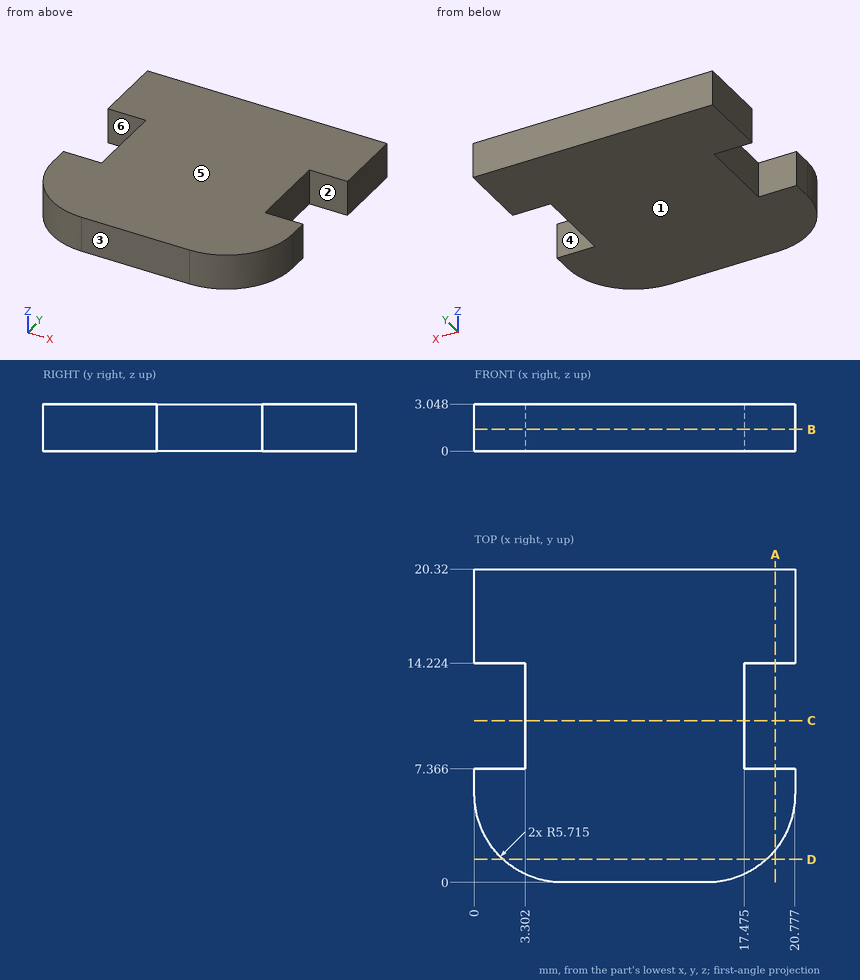
Check sheet for the drawn part. Datum: minimum x, y, z corner. Units: mm. A direction names the side the tool comes from. Give positions to 0.01 mm unless a question says otherwise; leave off trailing zeros. Write each loop counter-clockwise with the first axis right and the second up, starting at its lowest first coordinate (ties: lowest second). Pieces come first, ordered by that corner, then holes. Notation, with made-up numbers: M 10,50.25 L 60,50.25 A11 ccw 60,57.25 Z; hole C -7,-13.75 d2. An arc over 180 degrees is marked long. Write item = value, one per line.
(1) Sectioned sample at C-C (y = 10.5). Record the cut outline in (x, z) (1 decimal), then the cut area to 3 significant figures.
Found:
outline = M 3.3,0 L 17.5,0 L 17.5,3 L 3.3,3 Z
area = 43.2 mm2
(2) Access from +Z, -Z, +X, -X, +Y, -Y to the whole of each face (thin tool, end or side, straight path). Record for the marked faces 4, 5 and 6.
Found:
face_4 = +Z, -Z, +X
face_5 = +Z, +X, -X, +Y, -Y
face_6 = +Z, -Z, -X
(3) Go/stop test with a flat-tipped pin: pin 1 Ø1.5 at (x, z) = (19.5, 1.5) entering from -Y. Record where the tip stops, or that it passes through.
Found:
pin_1 = 1.35
(4) Draft check along Y on the marked faces 1, 2 and 3. Enter one of: released by +Y, released by -Y, zero draft, split by the parting line, or undercut.
Found:
face_1 = zero draft
face_2 = undercut
face_3 = released by -Y
(5) Sectioned sample at B-B (z = 1.4). Record the cut outline in (x, y) (1 decimal), then the cut area to 3 significant figures.
Found:
outline = M 0,5.7 A5.7 ccw 5.7,0 L 15.1,0 A5.7 ccw 20.8,5.7 L 20.8,7.4 L 17.5,7.4 L 17.5,14.2 L 20.8,14.2 L 20.8,20.3 L 0,20.3 L 0,14.2 L 3.3,14.2 L 3.3,7.4 L 0,7.4 Z
area = 363 mm2
(6) Material ranges on line 1 (X direction, y = 8, z = 2.2) (1 decimal); line 2 (Y direction, x = 19, z = 2.4) (1 decimal); line 3 (Y direction, x = 3.25, z = 2), recorded low to high.
Found:
line_1 = 3.3 to 17.5
line_2 = 1.6 to 7.4, 14.2 to 20.3
line_3 = 0.56 to 7.37, 14.22 to 20.32
(7) Sectioned sample at D-D (y = 1.5). Record the cut outline in (x, z).
Found:
outline = M 1.86,0 L 18.92,0 L 18.92,3.05 L 1.86,3.05 Z
(8) Sectioned sample at A-A (x = 19.5). Record the cut outline in (y, z).
Found:
outline = M 2.11,0 L 7.37,0 L 7.37,3.05 L 2.11,3.05 Z; M 14.22,0 L 20.32,0 L 20.32,3.05 L 14.22,3.05 Z
